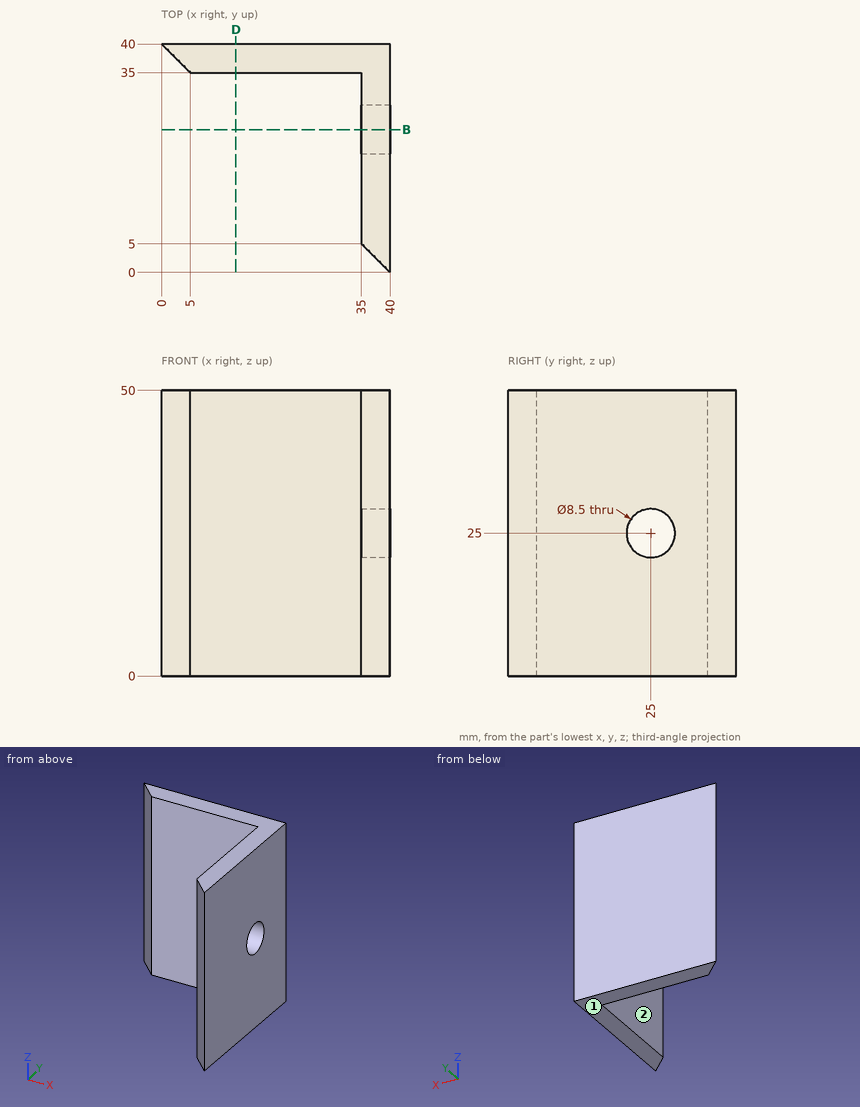
Could you check a few things on this drawing? It's one solid part, dimensions in mm from its lowest x, y, z. A direction names the side the tool comes from. Give positions to 0.01 mm unless a question says otherwise; leave off trailing zeros. Order: outer loops, then holes, each group sorted by start corner. A loop starts at its lowest first (then second) coordinate and runs counter-clockwise, first axis right, second up. Notation, with made-up numbers: (62.5, 71.25) -> (71.5, 71.25) arc R34 cw to (71.5, 106.25) -> close; hole circle Ø1 at (86.5, 10). An arc over 180 degrees is marked (long way). Answer in a Markdown table with one row per item. Add a question column.
Item 1: Imagine slicing it at B-B (y = 25). List the corners of the cut face in (x, z) for me.
Item 2: I'm going to push flat-ended pins straight in: P1, Ø5, axis at y = 25, z = 25, coming from the +X side; P2, Ø10, axis at y = 11, z = 42, coming from the -X side. Where does each tip first touch, or does it pass through?
Item 3: Imagine slicing it at D-D (x = 13). List the corners of the cut face in (y, z) for me.
Item 4: Please list where these lines run through material, in increasing order: probe 1 along Z at (x, y) = (37.65, 25); probe 2 along Y at (x, z) = (14.5, 9).
Item 5: For the marked faces 1 and 2, which set-ups out of +Z, -Z, +X, -X, +Y, -Y let a thin tool reach every point of the face, with its end or its side?
Result:
| question | item | result |
|---|---|---|
| 1 | outline | (35, 0) -> (40, 0) -> (40, 20.75) -> (35, 20.75) -> close; (35, 29.25) -> (40, 29.25) -> (40, 50) -> (35, 50) -> close |
| 2 | P1 | through |
| 2 | P2 | x = 35 |
| 3 | outline | (35, 0) -> (40, 0) -> (40, 50) -> (35, 50) -> close |
| 4 | probe 1 | 0 to 20.75, 29.25 to 50 |
| 4 | probe 2 | 35 to 40 |
| 5 | face 1 | -Z, +X, -X, +Y, -Y |
| 5 | face 2 | +Z, -Z, -X, -Y |
